```python
from build123d import *

# Parameters (mm, degrees)
SKETCH_W   = 110
SKETCH_H   = 117
SKETCH_R   = 8
SKETCH_W_2 = 80
SKETCH_H_2 = 45
PAD_DEPTH  = 4


with BuildPart() as part:
    # Sketch → Pad (new body)
    with BuildSketch(Plane.XY):
        Rectangle(SKETCH_W, SKETCH_H)
        with Locations((0, -38.5)):
            Circle(SKETCH_R, mode=Mode.SUBTRACT)
        with Locations((-28, -38.5)):
            Circle(SKETCH_R, mode=Mode.SUBTRACT)
        with Locations((28, -38.5)):
            Circle(SKETCH_R, mode=Mode.SUBTRACT)
        with Locations((0, 22.5)):
            Rectangle(SKETCH_W_2, SKETCH_H_2, mode=Mode.SUBTRACT)
    extrude(amount=PAD_DEPTH)


solid = part.part
```
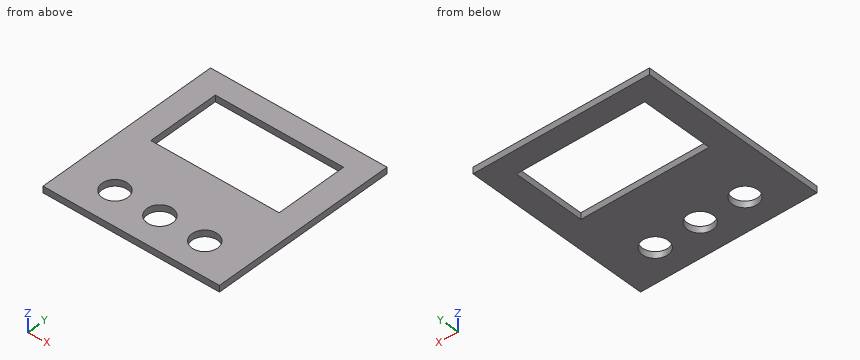
Work out the finished part from the listing and answer in its coordinate system (mm). Give positions to 0.01 mm unless a question says otherwise; leave off trailing zeros. Order: outer loops, then holes, each group sorted by start corner. A loop starts at its lowest first (then second) coordinate and runs counter-clockwise, first axis right, second up. Notation, with made-up numbers: (78, 77.25) - (116, 77.25) arc R25 cw to (116, 97.25) - close; hole circle Ø11 at (36, -25). An arc over 180 degrees is marked (long way). One line per item, written item: value. Start each with the question number.
1. Consider line 1 (Y direction, x = 0, z = 2.9); line 2 (X direction, y = 29.5, z = 1.25); line 3 (Y direction, x = -2, z = 0.8). Determine where each line is inside the solid, lowest interval first.
2. This flat-tipped pin is pushed along its axis until it touches: pin 1 Ø13 at (x, y) = (0, -38.5) entering from +Z. Where does it stop, or does it pass through?
3. Section A-A, the plane x = -38.5 is taken. Write down the section's boundary in (y, z), then the cut area to 3 significant figures.
4. Section B-B, the plane y = -38.5 is taken. Write down the section's boundary in (x, z), then the cut area to 3 significant figures.
5. Section D-D, the plane x = 0 is taken. Write down the section's boundary in (y, z), then the cut area to 3 significant figures.
6. Section C-C, the plane z = 0.75 is taken. Write down the section's boundary in (x, y).
Filled sheet:
1. line 1: -58.5 to -46.5, -30.5 to 0, 45 to 58.5
1. line 2: -55 to -40, 40 to 55
1. line 3: -58.5 to -46.25, -30.75 to 0, 45 to 58.5
2. pin 1: through
3. outline: (-58.5, 0) - (0, 0) - (0, 4) - (-58.5, 4) - close; (45, 0) - (58.5, 0) - (58.5, 4) - (45, 4) - close
3. area: 288 mm²
4. outline: (-55, 0) - (-36, 0) - (-36, 4) - (-55, 4) - close; (-20, 0) - (-8, 0) - (-8, 4) - (-20, 4) - close; (8, 0) - (20, 0) - (20, 4) - (8, 4) - close; (36, 0) - (55, 0) - (55, 4) - (36, 4) - close
4. area: 248 mm²
5. outline: (-58.5, 0) - (-46.5, 0) - (-46.5, 4) - (-58.5, 4) - close; (-30.5, 0) - (0, 0) - (0, 4) - (-30.5, 4) - close; (45, 0) - (58.5, 0) - (58.5, 4) - (45, 4) - close
5. area: 224 mm²
6. outline: (-55, -58.5) - (55, -58.5) - (55, 58.5) - (-55, 58.5) - close; hole (-40, 0) - (40, 0) - (40, 45) - (-40, 45) - close; hole circle Ø16 at (-28, -38.5); hole circle Ø16 at (0, -38.5); hole circle Ø16 at (28, -38.5)
